Can you work these out from the model? Positions are in its coordinate system, mm. Face numbers are marked on the shaded views. Give positions to 0.01 mm unless a question says otherwise; leave off trailing zeros. Loops run counter-clockwise (first coordinate to the right, second up) from the corner with the lowest first, then second, coordinate; pieces in that order, holes last. Notation, with made-up numbers: M -21,61 L 35,61 A17 ccw 35,67 Z; hole C 31,-21.5 d5. An arc over 180 degrees is marked long. Answer as a JSON object with one key per item and string values.
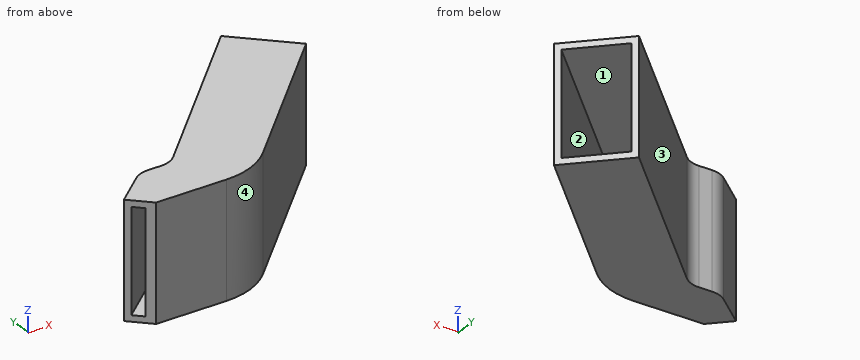
```python
from build123d import *

# Parameters (mm, degrees)
F1_DEPTH = 24
F2_R     = 15.1
F3_T     = -1.3
F5_DEPTH = 24.001
F6_R     = 5


with BuildPart() as f1:
    # F0 (on Top) → F1 (new body)
    with BuildSketch(Plane.XY):
        Polygon((-26.533620432, -25.4221484065), (-34.1206180562, -31.880568529), (-34.1206180562, -35.880568529), (-9.1206180562, -35.880568529), (23.5945900374, -3.1653604354), (12.9879883196, 7.4412412824), (-19.8754013693, -25.4221484065), align=None)
    extrude(amount=F1_DEPTH)

    # F2
    f2_edges = [f1.edges().sort_by_distance(p)[0] for p in [
        (-9.120618, -35.880569, 12),
    ]]
    fillet(f2_edges, radius=F2_R)

    # F3
    f3_openings = [f1.faces().sort_by_distance(p)[0] for p in [
        (-34.120618, -33.880569, 12),
        (18.291289, 2.13794, 12),
    ]]
    offset(amount=F3_T, openings=f3_openings, kind=Kind.INTERSECTION)

    # F4 (on face) → F5 (cut, through all)
    with BuildSketch(Plane.XY.offset(24)):
        Polygon((-30.1206180562, -35.880568529), (-34.1206180562, -31.880568529), (-34.1206180562, -35.880568529), align=None)
    extrude(amount=-F5_DEPTH, mode=Mode.SUBTRACT)

    # F6
    f6_edges = [f1.edges().sort_by_distance(p)[0] for p in [
        (-26.53362, -25.422148, 12),
        (-19.875401, -25.422148, 12),
    ]]
    fillet(f6_edges, radius=F6_R)


solid = f1.part
```
1) If we mould it in two halves opening along Y, with no side actions, what happens to the marked faces 1, 2, 3 and 4? For each: +Y half, -Y half, draft (parallel to the pull), parting line (faces both ways), or undercut.
Answer list:
{"face 1": "undercut", "face 2": "undercut", "face 3": "+Y half", "face 4": "-Y half"}
2) Suppose I cut it at D-D, the plane x = 16.5. Write out the boundary of the cut face in (y, z), and give its area (3 significant figures).
Answer list:
{"outline": "M -10.26,0 L 3.93,0 L 3.93,1.3 L -8.42,1.3 L -8.42,22.7 L 3.93,22.7 L 3.93,24 L -10.26,24 Z", "area": "76.2 mm^2"}
3) Suppose I cut it at A-A, the plane z = 10. Write out the boundary of the cut face in (x, y).
Answer list:
{"outline": "M -34.12,-31.88 L -33.2,-32.8 L -26.06,-26.72 L -19.34,-26.72 L 13.91,6.52 L 12.99,7.44 L -18.41,-23.96 A5 cw -21.95,-25.42 L -24.69,-25.42 A5 ccw -27.93,-26.61 Z; M -31.42,-34.58 L -30.12,-35.88 L -15.38,-35.88 A15.1 ccw -4.7,-31.46 L 23.59,-3.17 L 22.68,-2.25 L -5.62,-30.54 A13.8 cw -15.38,-34.58 Z"}
4) Will these pins go through, and if not, where does the flat tip stop? pin 1 Ø5 at (y, z) = (-18.5, 20) entering from +X; pin 2 Ø1.5 at (x, z) = (-2.5, 7.5) entering from +Y; pin 3 Ø2 at (x, z) = (16, 7.5) entering from -Y.
Answer list:
{"pin 1": "x = 10.76", "pin 2": "y = -7.3", "pin 3": "y = -11.76"}
5) Suppose I cut it at B-B, the plane y = -5.5. Write out the boundary of the cut face in (x, z), and give its area (3 significant figures).
Answer list:
{"outline": "M 0.05,0 L 21.26,0 L 21.26,24 L 0.05,24 Z; hole M 1.89,1.3 L 19.42,1.3 L 19.42,22.7 L 1.89,22.7 Z", "area": "134 mm^2"}
6) Suppose I cut it at C-C, the plane x = -9. Write out the boundary of the cut face in (y, z).
Answer list:
{"outline": "M -34.47,0 L -14.55,0 L -14.55,24 L -34.47,24 Z; hole M -33.02,1.3 L -16.39,1.3 L -16.39,22.7 L -33.02,22.7 Z"}
7) Please list where these lines run through material, in increasing order: line 1 along Z through (x, y) = (8.5, -10); line 2 along Y through (x, z) = (-23, 2.5); line 3 along Y through (x, z) = (-3.5, 22). Write a range as from..to.
Answer list:
{"line 1": "0..1.3, 22.7..24", "line 2": "-35.88..-34.58, -26.72..-25.42", "line 3": "-30.26..-28.42, -10.89..-9.05"}
